from build123d import *

# Parameters (mm, degrees)
SKETCH1_R                      = 2
BOSS_EXTRUDE1_DEPTH            = 4
SKETCH2_W                      = 12
SKETCH2_H                      = 5
BOSS_EXTRUDE2_DEPTH            = 37
SKETCH3_R                      = 2
SKETCH3_W                      = 12
SKETCH3_H                      = 5
BOSS_EXTRUDE3_DEPTH            = 4
FILLET1_R                      = 3
CUT_EXTRUDE1_REACH             = 56.891
SKETCH4_W                      = 12
SKETCH4_H                      = 19.420745895
CUT_EXTRUDE1_DIRECTION_2_DEPTH = 10


with BuildPart() as part:
    # Sketch1 → Boss-Extrude1 (new body)
    with BuildSketch(Plane(origin=(0, 0, 0), x_dir=(1, 0, 0), z_dir=(0, 1, 0))):
        with BuildLine():
            ThreePointArc((6, 30), (0, 36), (-6, 30))
            Line((-6, 30), (-6, 0))
            ThreePointArc((-6, 0), (0, -6), (6, 0))
            Line((6, 0), (6, 30))
        make_face()
        with Locations(Location((0, 30, 0), (0, 0, 270))):
            Circle(SKETCH1_R, mode=Mode.SUBTRACT)
        with Locations(Location((0, 0, 0), (0, 0, 270))):
            Circle(SKETCH1_R, mode=Mode.SUBTRACT)
    extrude(amount=BOSS_EXTRUDE1_DEPTH)

    # Sketch2 → Boss-Extrude2 (add)
    with BuildSketch(Plane(origin=(0, 4, 0), x_dir=(1, 0, 0), z_dir=(0, 1, 0))):
        with Locations((0, 15)):
            Rectangle(SKETCH2_W, SKETCH2_H)
    extrude(amount=BOSS_EXTRUDE2_DEPTH)

    # Sketch3 → Boss-Extrude3 (add)
    # profile 1 of 2: a face of its own
    with BuildSketch(Plane(origin=(0, 41, 0), x_dir=(1, 0, 0), z_dir=(0, 1, 0))):
        with BuildLine():
            Line((6, 17.5), (6, 30))
            ThreePointArc((6, 30), (0, 36), (-6, 30))
            Line((-6, 30), (-6, 17.5))
            Line((-6, 17.5), (6, 17.5))
        make_face()
        with Locations(Location((0, 30, 0), (0, 0, 270))):
            Circle(SKETCH3_R, mode=Mode.SUBTRACT)
    # profile 2 of 2: a face of its own
    with BuildSketch(Plane(origin=(0, 41, 0), x_dir=(1, 0, 0), z_dir=(0, 1, 0))):
        with Locations((0, 15)):
            Rectangle(SKETCH3_W, SKETCH3_H)
    extrude(amount=BOSS_EXTRUDE3_DEPTH)

    # Fillet1
    fillet1_edges = [part.edges().sort_by_distance(p)[0] for p in [
        (0, 4, -17.5),
        (0, 41, -17.5),
        (0, 4, -12.5),
    ]]
    fillet(fillet1_edges, radius=FILLET1_R)

    # Sketch4 → Cut-Extrude1 (cut, up to next)
    with BuildSketch(Plane(origin=(0, 4, 0), x_dir=(1, 0, 0), z_dir=(0, 1, 0)), mode=Mode.PRIVATE) as cut_extrude1_sk1:
        with Locations((0, 27.210372948)):
            Rectangle(SKETCH4_W, SKETCH4_H)
    cut_extrude1_tool1 = extrude(cut_extrude1_sk1.sketch, amount=-CUT_EXTRUDE1_REACH, mode=Mode.PRIVATE) & part.part
    add(cut_extrude1_tool1.solids().sort_by_distance((0, 4, -27.210373))[0], mode=Mode.SUBTRACT)

    # Sketch4 → Cut-Extrude1 direction 2 (cut)
    with BuildSketch(Plane(origin=(0, 4, 0), x_dir=(1, 0, 0), z_dir=(0, 1, 0))):
        with Locations((0, 27.210372948)):
            Rectangle(SKETCH4_W, SKETCH4_H)
    extrude(amount=CUT_EXTRUDE1_DIRECTION_2_DEPTH, mode=Mode.SUBTRACT)


solid = part.part
Could you check a few things on this model? Use its own coordinates, in mm. A direction names the side the tool comes from. Round coordinates to 2 decimals unless told otherwise and drop trailing zeros. Order: outer loops, then holes, each group sorted by start corner. A loop starts at its lowest first (then second) coordinate and runs counter-clockwise, first axis right, second up.
Q1. Imagine slicing it at A-A, the plane x = 0. List the corners of the cut face in (y, z) for me, then the cut area to 3 significant figures.
Geometry says:
outline: (0, -17.5) - (38, -17.5) arc R3 cw to (41, -20.5) - (41, -28) - (45, -28) - (45, -12.5) - (7, -12.5) arc R3 cw to (4, -9.5) - (4, -2) - (0, -2) - close; (0, 2) - (4, 2) - (4, 6) - (0, 6) - close; (41, -36) - (45, -36) - (45, -32) - (41, -32) - close
area: 345 mm2
Q2. Imagine slicing it at C-C, the plane x = -4.75. List the corners of the cut face in (y, z) for me, then the cut area to 3 significant figures.
Geometry says:
outline: (0, -17.5) - (38, -17.5) arc R3 cw to (41, -20.5) - (41, -33.67) - (45, -33.67) - (45, -12.5) - (7, -12.5) arc R3 cw to (4, -9.5) - (4, 3.67) - (0, 3.67) - close
area: 358 mm2
Q3. Please list where these lines run through material, in increasing order: probe 1 along X at (y, z) = (43.2, -30); probe 2 along Y at (x, z) = (3.5, 2); probe 3 along Z at (x, y) = (-5, 25).
Geometry says:
probe 1: x = -6 to -2, 2 to 6
probe 2: y = 0 to 4
probe 3: z = -17.5 to -12.5
Q4. Imagine slicing it at B-B, the plane z = -1. List the corners of the cut face in (x, y) for me, then the cut area to 3 significant figures.
Geometry says:
outline: (-6, 0) - (-1.73, 0) - (-1.73, 4) - (-6, 4) - close; (1.73, 0) - (6, 0) - (6, 4) - (1.73, 4) - close
area: 34.1 mm2
Q5. Which directions (+Z, -Z, +X, -X, +Y, -Y) give clear straight access to the entire face, cutting with the end or side of a thin tool? Please do faces 1 (the face through (0, 19, -17.5)), 2 (the face through (0, 4, -4)), 3 (the face through (0, 0, -6)).
Geometry says:
face 1: -Z, +X, -X, -Y
face 2: +Z, +X, -X, +Y
face 3: +Z, -Z, +X, -X, -Y
Q6. I'm going to push flat-ended pins straight in: P1, Ø3, axis at x = 0, z = -30, coming from the +Y side; P2, Ø2, axis at x = -3.5, y = 40, coming from the +Z side; P3, Ø5, axis at x = -4, y = 5, coming from the -Z side; P4, Ø3.5, axis at x = 0.5, z = -3.5, coming from the +Y side. Where does each tip first touch, or does it pass through?
Geometry says:
P1: passes through
P2: stops at z = -12.5
P3: stops at z = -17.5
P4: stops at y = 4
Q7. Thinking about a two-plate mould opening in Y: for faces 4 (the face through (0, 41, -27)), 5 (the face through (0.08, 4.9, -11.64)), 6 (the face through (0, 26, -12.5)), which applies, released by +Y, released by -Y, zero draft, split by the parting line, or undercut?
Geometry says:
face 4: released by -Y
face 5: released by +Y
face 6: zero draft
Q8. Imagine slicing it at D-D, the plane y = 18.5. List the corners of the cut face in (x, z) for me, then the cut area to 3 significant figures.
Geometry says:
outline: (-6, -17.5) - (6, -17.5) - (6, -12.5) - (-6, -12.5) - close
area: 60.0 mm2
